The figure shows three views and two pictorial views of one solid part (mm, origin at its lowest corner). Answer the questions. Round coordinates to 2 decimals unless told otherwise and drop trailing zeros. Order: outer loops, then holes, each group sorted by start corner. A loop starts at its lowest first (then second) coordinate and runs counter-clockwise, first axis right, second up. Notation, with made-up numbers: (-20, -40) - (32, -40) arc R32 cw to (32, -10) - close; hole circle Ø2 at (58, -17.5). An arc over 180 degrees is marked (long way). Use CSV: the item, a comma, the result in double quotes. Start each with the question number.
Item 1: Straight lines are drawn through the part: line 1 along X through (y, z) = (4, 258.5); line 2 along Z through (x, y) = (33, 4.75); line 3 along X through (y, z) = (1.25, 28). For each, find the intervals that lie inside material, in ascending order. Write a range as [from, to].
Item 2: Find section C-C, the plane y = 2.25. Give the vertices of the cut face in (x, z), plus the area to 3 significant figures.
Item 3: Find section B-B, the plane x = 68.5. Give the vertices of the cut face in (y, z), plus the area to 3 significant figures.
Item 4: Find section A-A, the plane z = 139.5. Give the vertices of the cut face in (x, y), plus the area to 3 significant figures.
Item 5: Flat-ended cylindrical pins translate along their axes: P1, Ø1.9, axis at y = 4.5, z = 224, coming from the -X side; P2, Ø8, axis at x = 160.5, z = 193, coming from the +Y side. Find the tip coordinate at first contact, or state that the pin passes through.
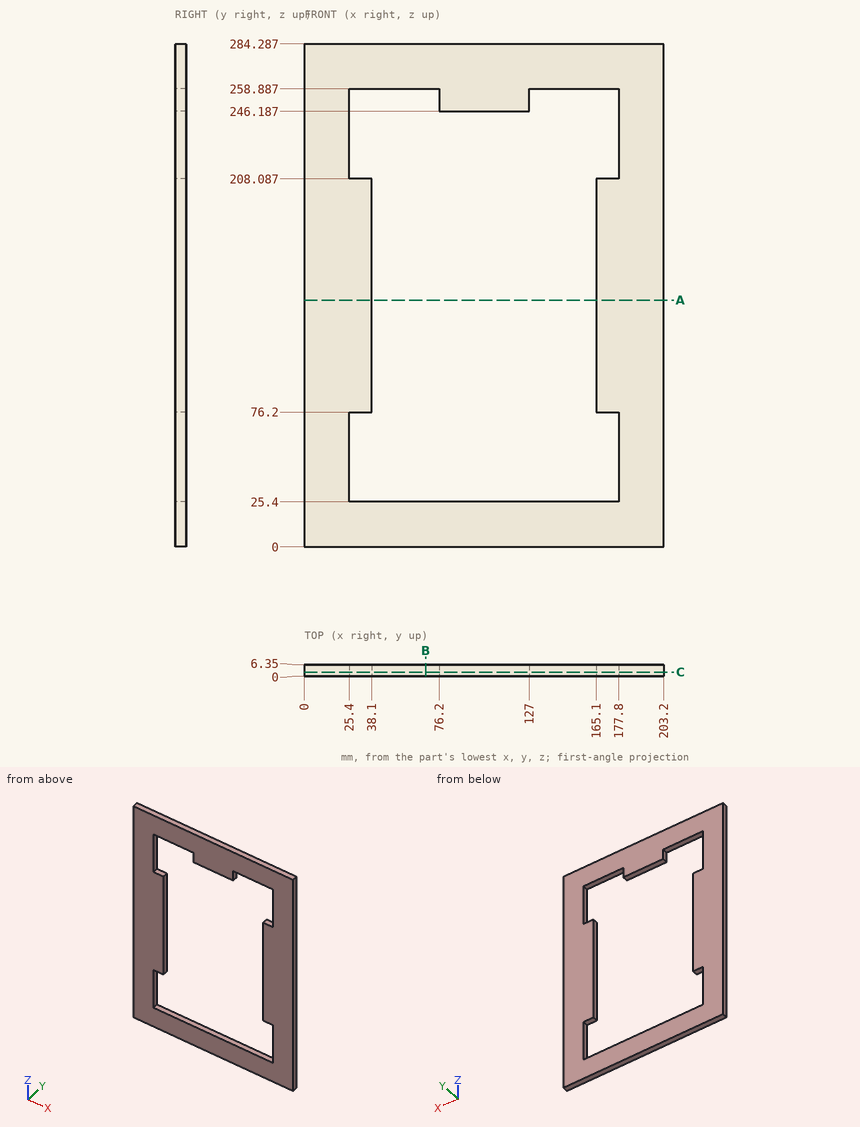
Worked out:
1,line 1,"x = [0, 25.4], [76.2, 127], [177.8, 203.2]"
1,line 2,"z = [0, 25.4], [76.2, 208.09], [258.89, 284.29]"
1,line 3,"x = [0, 25.4], [177.8, 203.2]"
2,outline,"(0, 0) - (203.2, 0) - (203.2, 284.29) - (0, 284.29) - close; hole (25.4, 25.4) - (177.8, 25.4) - (177.8, 76.2) - (165.1, 76.2) - (165.1, 208.09) - (177.8, 208.09) - (177.8, 258.89) - (127, 258.89) - (127, 246.19) - (76.2, 246.19) - (76.2, 258.89) - (25.4, 258.89) - (25.4, 208.09) - (38.1, 208.09) - (38.1, 76.2) - (25.4, 76.2) - close"
2,area,"26,200 mm²"
3,outline,"(0, 0) - (6.35, 0) - (6.35, 25.4) - (0, 25.4) - close; (0, 258.89) - (6.35, 258.89) - (6.35, 284.29) - (0, 284.29) - close"
3,area,"323 mm²"
4,outline,"(0, 0) - (38.1, 0) - (38.1, 6.35) - (0, 6.35) - close; (165.1, 0) - (203.2, 0) - (203.2, 6.35) - (165.1, 6.35) - close"
4,area,"484 mm²"
5,P1,"stops at x = 0"
5,P2,"passes through"
